CAD build for the part. Positions are in the model's coordinates, mm. A direction names the side the tool comes from. Coordinates: 2 decimals unless noted, no trailing zeros. Loops run counter-clockwise (first coordinate to the right, second up) from the corner with the lowest first, then second, coordinate; pieces in that order, holes last. Notation, with made-up numbers: (24.5, -3) - (81.5, -3) arc R21 ccw to (81.5, 21) - close; hole circle Ø3 at (78, -6). An arc over 180 degrees is marked (long way). Put each result on its own line as item: value.
```python
from build123d import *

# Parameters (mm, degrees)
SKETCH1_W                                  = 406.4
SKETCH1_H                                  = 152.4
SKETCH1_W_2                                = 381
SKETCH1_H_2                                = 127
BOSS_EXTRUDE1_DEPTH                        = 12.7
SKETCH2_W                                  = 12.7
SKETCH2_H                                  = 12.7
BOSS_EXTRUDE2_DEPTH                        = 146.05
MIRROR1_AT_THE_SECOND_PLANE_COPY_1_SKETC_W = 12.7
MIRROR1_AT_THE_SECOND_PLANE_COPY_1_SKETC_H = 12.7
MIRROR1_AT_THE_SECOND_PLANE_COPY_1_DEPTH   = 146.05
SKETCH3_W                                  = 406.4
SKETCH3_H                                  = 152.4
SKETCH3_W_2                                = 381
SKETCH3_H_2                                = 127
BOSS_EXTRUDE3_DEPTH                        = 6.35
SKETCH6_W                                  = 12.7
SKETCH6_H                                  = 12.7
CUT_EXTRUDE1_DEPTH                         = 381
BOSS_EXTRUDE5_DEPTH                        = 381
CUT_EXTRUDE3_DEPTH                         = 262.586090035
LOFT2_START                                = -63.5
LOFT2_DEPTH                                = 127
LOFT3_START                                = -63.5
LOFT3_DEPTH                                = 127


# Read off the part's stored shape, not the designer's step: Loft2, Loft3
with BuildPart() as part:
    # Sketch1 → Boss-Extrude1 (new body)
    with BuildSketch(Plane(origin=(0, 0, 0), x_dir=(1, 0, 0), z_dir=(0, 1, 0))):
        Rectangle(SKETCH1_W, SKETCH1_H)
        Rectangle(SKETCH1_W_2, SKETCH1_H_2, mode=Mode.SUBTRACT)
    extrude(amount=BOSS_EXTRUDE1_DEPTH)

    # Sketch2 → Boss-Extrude2 (add)
    with BuildSketch(Plane(origin=(0, 12.7, 0), x_dir=(1, 0, 0), z_dir=(0, 1, 0))):
        with Locations((-196.85, -69.85)):
            Rectangle(SKETCH2_W, SKETCH2_H)
    boss_extrude2 = extrude(amount=BOSS_EXTRUDE2_DEPTH)

    # Mirror1: Boss-Extrude2 across plane
    add(boss_extrude2.mirror(Plane(origin=(0, 0, 0), x_dir=(0, 0, 1), z_dir=(1, 0, 0))))

    # Mirror1 at the second plane: Boss-Extrude2 across plane
    add(boss_extrude2.mirror(Plane.XY))

    # Mirror1 at the second plane copy 1 sketc → Mirror1 at the second plane copy 1 (add)
    with BuildSketch(Plane(origin=(0, 12.7, 0), x_dir=(-1, 0, 0), z_dir=(0, 1, 0))):
        with Locations((-196.85, -69.85)):
            Rectangle(MIRROR1_AT_THE_SECOND_PLANE_COPY_1_SKETC_W, MIRROR1_AT_THE_SECOND_PLANE_COPY_1_SKETC_H)
    extrude(amount=MIRROR1_AT_THE_SECOND_PLANE_COPY_1_DEPTH)

    # Sketch3 → Boss-Extrude3 (add)
    with BuildSketch(Plane(origin=(0, 158.75, 0), x_dir=(1, 0, 0), z_dir=(0, 1, 0))):
        Rectangle(SKETCH3_W, SKETCH3_H)
        Rectangle(SKETCH3_W_2, SKETCH3_H_2, mode=Mode.SUBTRACT)
    extrude(amount=-BOSS_EXTRUDE3_DEPTH)

    # Sketch6 → Cut-Extrude1 (cut)
    with BuildSketch(Plane.ZY.offset(-190.5)):
        with Locations((-69.85, 6.35)):
            Rectangle(SKETCH6_W, SKETCH6_H)
    extrude(amount=CUT_EXTRUDE1_DEPTH, mode=Mode.SUBTRACT)

    # Sketch4 → Boss-Extrude5 (add)
    with BuildSketch(Plane.ZY.offset(-190.5)):
        Polygon((-63.5, 0), (63.5, 0), (63.5, 12.7), (-63.5, 1.27), align=None)
    extrude(amount=BOSS_EXTRUDE5_DEPTH)

    # Sketch10 → Cut-Extrude3 (cut, through all)
    with BuildSketch(Plane(origin=(0, 12.7, 0), x_dir=(1, 0, 0), z_dir=(0, 1, 0))):
        Polygon((-190.5, -63.5), (-190.5, 63.5), (-50.8, 63.5), align=None)
        Polygon((190.5, -63.5), (190.5, 63.5), (50.8, 63.5), align=None)
    extrude(amount=-CUT_EXTRUDE3_DEPTH, mode=Mode.SUBTRACT)

    # Loft2 outline → Loft2 (add)
    with BuildSketch(Plane.XY.offset(LOFT2_START)):
        Polygon((49, 1.122727273), (49, 0), (190.5, 0), (190.5, 12.7), (50.8, 1.27), align=None)
    extrude(amount=LOFT2_DEPTH)

    # Loft3 outline → Loft3 (add)
    with BuildSketch(Plane.XY.offset(LOFT3_START)):
        Polygon((-190.5, 12.7), (-190.5, 0), (-49, 0), (-49, 1.122727273), (-50.8, 1.27), align=None)
    extrude(amount=LOFT3_DEPTH)


solid = part.part
```
Q1. Slice it at A-A, the plane z = 28.5. Give the cut face in (x, y).
Determined:
outline: (-203.2, 0) - (203.2, 0) - (203.2, 12.7) - (190.5, 12.7) - (152, 9.55) - (-152, 9.55) - (-190.5, 12.7) - (-203.2, 12.7) - close; (-203.2, 152.4) - (-190.5, 152.4) - (-190.5, 158.75) - (-203.2, 158.75) - close; (190.5, 152.4) - (203.2, 152.4) - (203.2, 158.75) - (190.5, 158.75) - close
Q2. Slice it at B-B, the plane x = 174. Give the cut face in (y, z).
Determined:
outline: (0, -63.5) - (11.35, -63.5) - (11.35, 48.5) - (12.7, 63.5) - (12.7, 76.2) - (0, 76.2) - close; (152.4, -76.2) - (158.75, -76.2) - (158.75, -63.5) - (152.4, -63.5) - close; (152.4, 63.5) - (158.75, 63.5) - (158.75, 76.2) - (152.4, 76.2) - close
Q3. Pin check, flat tips, straight feed: pin 1 Ø8 at (x, z) = (80, 52.5) entering from -Y; pin 2 Ø12 at (x, z) = (108.5, -14.5) entering from +Y; pin 3 Ø14 at (x, y) = (-20.5, 7.5) entering from -Z; pin 4 Ø10 at (x, z) = (126.5, 0.5) entering from +Y. Stop position of each tip, or through.
Determined:
pin 1: y = 0
pin 2: y = 6.48
pin 3: z = -63.5
pin 4: y = 7.87
Q4. Mould opens along X. For faces 1 (the flat face through (1, 8, 76.2)), 2 (the flat face through (2.667, 8.335, 15)), 3 (the flat face through (203.2, 8, 0)) say: +X half, -X half, draft (parallel to the pull), parting line (faces both ways), or undercut.
Determined:
face 1: draft
face 2: undercut
face 3: +X half
Q5. Wall check: L1, parallel to X at y = 138.5, z = 67; L2, parallel to Y at x = -50, z = -69.5; L3, parallel to Y at x = 58, z = 36.5. Give the ranges that are in metal, low to high. Write a range as from..to.
Determined:
L1: -203.2..-190.5, 190.5..203.2
L2: 152.4..158.75
L3: 0..10.27
Q6. Slice it at D-D, the plane z = 57.5. Give the cut face in (x, y).
Determined:
outline: (-203.2, 0) - (203.2, 0) - (203.2, 12.7) - (190.5, 12.7) - (183.9, 12.16) - (-183.9, 12.16) - (-190.5, 12.7) - (-203.2, 12.7) - close; (-203.2, 152.4) - (-190.5, 152.4) - (-190.5, 158.75) - (-203.2, 158.75) - close; (190.5, 152.4) - (203.2, 152.4) - (203.2, 158.75) - (190.5, 158.75) - close
Q7. Tool access for faces 4 (the flat face through (-3, 1, -63.5)), 5 (the flat face through (-3, 152.4, -70)), 6 (the flat face through (-197, 82, -63.5)): list every direction of +Z, -Z, +X, -X, +Y, -Y with a clear straight run to the whole face (end or side of a thin tool).
Determined:
face 4: -Z, -Y
face 5: +Z, -Z, -Y
face 6: +X, -X
Q8. Slice it at C-C, the plane y = 82.5. Give the cut face in (x, z).
Determined:
outline: (-203.2, -76.2) - (-190.5, -76.2) - (-190.5, -63.5) - (-203.2, -63.5) - close; (-203.2, 63.5) - (-190.5, 63.5) - (-190.5, 76.2) - (-203.2, 76.2) - close; (190.5, -76.2) - (203.2, -76.2) - (203.2, -63.5) - (190.5, -63.5) - close; (190.5, 63.5) - (203.2, 63.5) - (203.2, 76.2) - (190.5, 76.2) - close
